Answer from the drawing. Dimensions are ordinates in mm from the lowest x, y and z of the part. Give positions to 0.01 mm unless a question says otherwise; leave off trailing zeros. Order: outer loops, then holes, each group sorted by start corner. A loop starts at its lowest first (then second) coordinate and runs counter-clockwise, first axis right, second up.
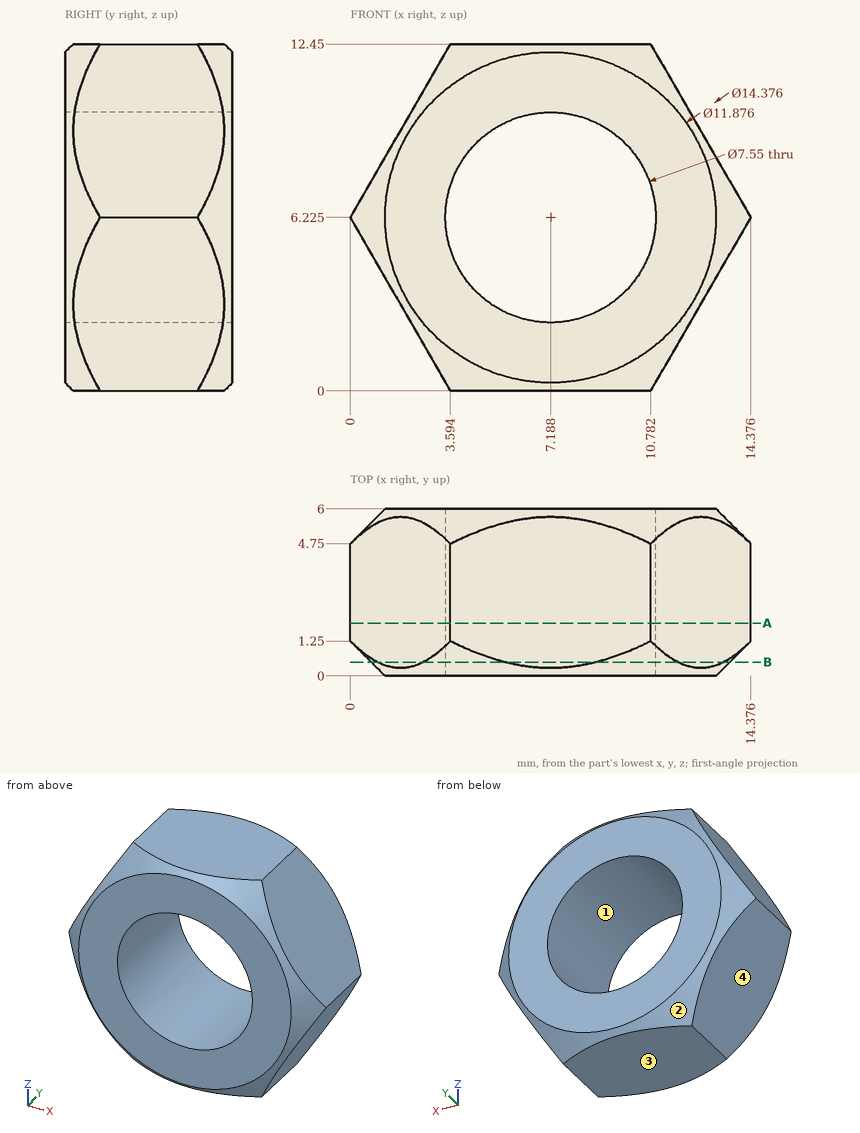
1) The part is cut by section B-B on y = 0.5. Determine the outline of the cut face in (x, z) (3 decimals), and give its area (3 significant figures).
Final values:
outline: (0.976, 4.535) - (2.618, 1.69) arc R6.438 ccw to (5.546, 0) - (8.83, 0) arc R6.438 ccw to (11.758, 1.69) - (13.4, 4.535) arc R6.438 ccw to (13.4, 7.915) - (11.758, 10.76) arc R6.438 ccw to (8.83, 12.45) - (5.546, 12.45) arc R6.438 ccw to (2.618, 10.76) - (0.976, 7.915) arc R6.438 ccw to start; hole circle Ø7.55 at (7.188, 6.225)
area: 82.6 mm2
2) For a pull along X with two mould halves and no side action, classify the marked faces 1, 2, 3 and 4 as released by +X, released by -X, zero draft, split by the parting line, or undercut.
Final values:
face 1: undercut
face 2: split by the parting line
face 3: zero draft
face 4: released by -X
3) The part is cut by section A-A on y = 1.9. Determine the outline of the cut face in (x, z) (3 decimals).
Final values:
outline: (0, 6.225) - (3.594, 0) - (10.782, 0) - (14.376, 6.225) - (10.782, 12.45) - (3.594, 12.45) - close; hole circle Ø7.55 at (7.188, 6.225)
4) Consider L1, parallel to Z at x = 8.25, y = 1.25; L2, parallel to Z at x = 4.5, y = 0.8; L3, parallel to X at y = 3.95, z = 4.5. Determine where each line is inside the solid, lowest interval first.
Final values:
L1: z = 0 to 2.6, 9.85 to 12.45
L2: z = 0.05 to 3.57, 8.88 to 12.4
L3: x = 1 to 3.83, 10.55 to 13.38
5) Given pin 1 (6 mm diameter, centred on x = 7.19, z = 6.22, fed in from -Y), flat-ended and moving along its own axis, determine where the tip first touches the part or whether it passes through.
Final values:
pin 1: passes through
